Design review of the part built by this model. Coordinates are the model's own, in mm. A direction names the side the tool comes from. Coordinates: 2 decimals unless noted, no trailing zeros. Write each loop counter-clockwise with the first axis right and the second up, starting at its lowest first coordinate (ties: lowest second). Pieces come first, ordered by that corner, then holes. Notation, with made-up numbers: (68.25, 6) - (80.25, 6) arc R35 ccw to (80.25, 43) - close; hole circle Ø5 at (36.5, 41). An arc over 180 degrees is marked (long way). Answer as a JSON object with one key per item and string values.
```python
from build123d import *

# Parameters (mm, degrees)
BOSS_EXTRUDE1_DEPTH = 10
CUT_EXTRUDE1_REACH  = 9
SKETCH2_W           = 4
SKETCH2_H           = 5.5
CUT_EXTRUDE2_REACH  = 6
SKETCH3_R           = 1.5


with BuildPart() as part:
    # Sketch1 → Boss-Extrude1 (new body)
    with BuildSketch(Plane.XY):
        Polygon((0, 0), (0, 10), (7, 10), (7, 3.5), (5.5, 0), align=None)
    extrude(amount=BOSS_EXTRUDE1_DEPTH)

    # Sketch2 → Cut-Extrude1 (cut, up to next)
    with BuildSketch(Plane(origin=(7, 0, 0), x_dir=(0, 0, -1), z_dir=(1, 0, 0)), mode=Mode.PRIVATE) as cut_extrude1_sk1:
        with Locations((-7.5, 6.75)):
            Rectangle(SKETCH2_W, SKETCH2_H)
    cut_extrude1_tool1 = extrude(cut_extrude1_sk1.sketch, amount=-CUT_EXTRUDE1_REACH, mode=Mode.PRIVATE) & part.part
    add(cut_extrude1_tool1.solids().sort_by_distance((7, 6.75, 7.5))[0], mode=Mode.SUBTRACT)
    # Sketch2 → Cut-Extrude1 (cut, up to next)
    with BuildSketch(Plane(origin=(7, 0, 0), x_dir=(0, 0, -1), z_dir=(1, 0, 0)), mode=Mode.PRIVATE) as cut_extrude1_sk2:
        with Locations((-2.5, 6.75)):
            Rectangle(SKETCH2_W, SKETCH2_H)
    cut_extrude1_tool2 = extrude(cut_extrude1_sk2.sketch, amount=-CUT_EXTRUDE1_REACH, mode=Mode.PRIVATE) & part.part
    add(cut_extrude1_tool2.solids().sort_by_distance((7, 6.75, 2.5))[0], mode=Mode.SUBTRACT)

    # Sketch3 → Cut-Extrude2 (cut, up to next)
    with BuildSketch(Plane(origin=(0, 4, 0), x_dir=(1, 0, 0), z_dir=(0, 1, 0)), mode=Mode.PRIVATE) as cut_extrude2_sk1:
        with Locations((3.5, -2.5)):
            Circle(SKETCH3_R)
    cut_extrude2_tool1 = extrude(cut_extrude2_sk1.sketch, amount=-CUT_EXTRUDE2_REACH, mode=Mode.PRIVATE) & part.part
    add(cut_extrude2_tool1.solids().sort_by_distance((3.5, 4, 2.5))[0], mode=Mode.SUBTRACT)
    # Sketch3 → Cut-Extrude2 (cut, up to next)
    with BuildSketch(Plane(origin=(0, 4, 0), x_dir=(1, 0, 0), z_dir=(0, 1, 0)), mode=Mode.PRIVATE) as cut_extrude2_sk2:
        with Locations((3.5, -7.5)):
            Circle(SKETCH3_R)
    cut_extrude2_tool2 = extrude(cut_extrude2_sk2.sketch, amount=-CUT_EXTRUDE2_REACH, mode=Mode.PRIVATE) & part.part
    add(cut_extrude2_tool2.solids().sort_by_distance((3.5, 4, 7.5))[0], mode=Mode.SUBTRACT)


solid = part.part
```
(1) To check wall thickness, follow line 1 (Z direction, x = 3.75, y = 8.25); line 2 (Z direction, x = 3.5, y = 3.1); line 3 (Y direction, x = 0.5, z = 6). State the ranges of each line that lie inside material, in increasing order. Write a range as from..to.
Solved:
{"line 1": "z = 0..0.5, 4.5..5.5, 9.5..10", "line 2": "z = 0..1, 4..6, 9..10", "line 3": "y = 0..4, 9.5..10"}
(2) Tool access review of faces 1 (the face through (4.306, 2.028, 1.235)), 2 (the face through (4, 7, 9.5)), 3 (the face through (3, 10, 5)): name each direction out of +Z, -Z, +X, -X, +Y, -Y from which nothing blocks a thin tool from reaching the whole face with its end or side.
Solved:
{"face 1": "-Y", "face 2": "+X, -X", "face 3": "+Z, -Z, +X, -X, +Y"}
(3) Take a section at A-A, the plane y = 5.5. Write out the cut boundary in (x, z).
Solved:
{"outline": "(0, 0) - (7, 0) - (7, 0.5) - (0, 0.5) - close; (0, 4.5) - (7, 4.5) - (7, 5.5) - (0, 5.5) - close; (0, 9.5) - (7, 9.5) - (7, 10) - (0, 10) - close"}
(4) The part is to be moulded in two halves that separate along Z. For faces 4 (the face through (4, 9.5, 3)), 5 (the face through (4, 5, 0)), 6 (the face through (7, 7, 5)), say which applies: pulls with the +Z half, pulls with the -Z half, needs draft (parallel to the pull), parting line crosses it, or undercut.
Solved:
{"face 4": "undercut", "face 5": "pulls with the -Z half", "face 6": "needs draft"}
(5) For pin 1 (2.5 mm diameter, centred on x = 3.5, z = 7.5, fed in from -Y); pin 2 (1.6 mm diameter, centred on x = 4.5, y = 8, fed in from -Z), all flat-tipped, find the tip position at first contact; note any pin that passes through.
Solved:
{"pin 1": "stops at y = 9.5", "pin 2": "stops at z = 0"}
(6) Take a section at D-D, the plane z = 8.75. Write out the cut boundary in (x, y), and give its area (3 significant figures).
Solved:
{"outline": "(0, 0) - (2.67, 0) - (2.67, 4) - (0, 4) - close; (0, 9.5) - (7, 9.5) - (7, 10) - (0, 10) - close; (4.33, 0) - (5.5, 0) - (7, 3.5) - (7, 4) - (4.33, 4) - close", "area": "22.2 mm^2"}
(7) Take a section at C-C, the plane x = 1. Write out the cut boundary in (y, z), and give its area (3 significant figures).
Solved:
{"outline": "(0, 0) - (10, 0) - (10, 10) - (0, 10) - close; hole (4, 0.5) - (9.5, 0.5) - (9.5, 4.5) - (4, 4.5) - close; hole (4, 5.5) - (9.5, 5.5) - (9.5, 9.5) - (4, 9.5) - close", "area": "56.0 mm^2"}
(8) Take a section at B-B, the plane z = 7.5. Write out the cut boundary in (x, y).
Solved:
{"outline": "(0, 0) - (2, 0) - (2, 4) - (0, 4) - close; (0, 9.5) - (7, 9.5) - (7, 10) - (0, 10) - close; (5, 0) - (5.5, 0) - (7, 3.5) - (7, 4) - (5, 4) - close"}
